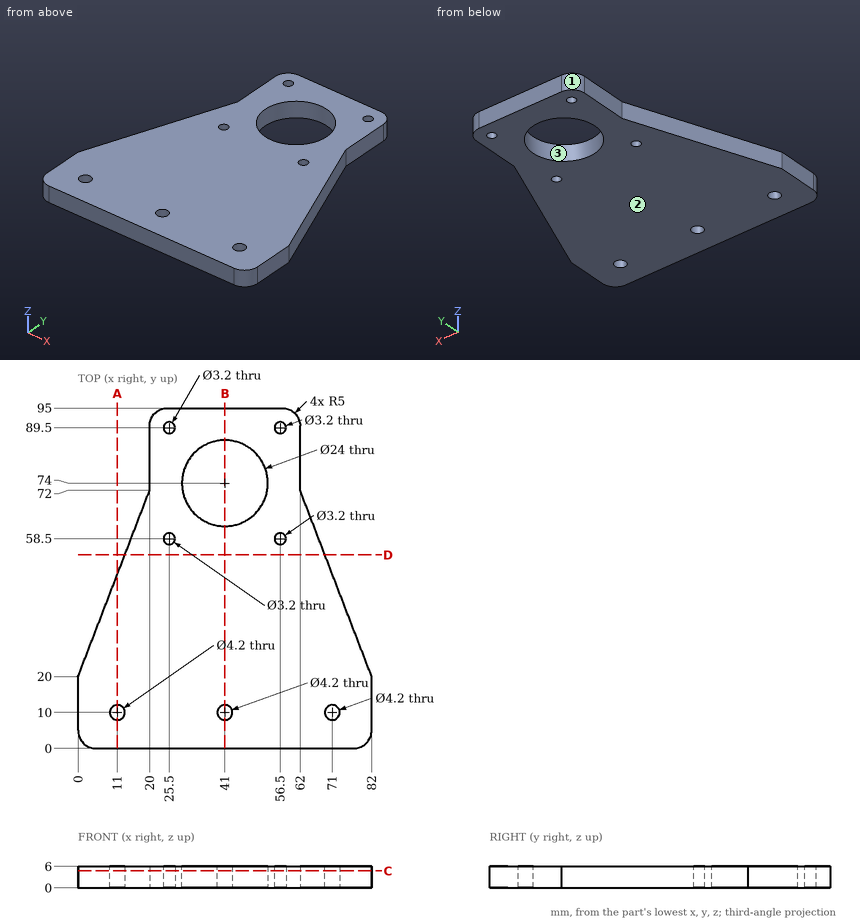
Here's the drawing with two shaded views (mm, measured from the low corner). I have some questions. Give positions to 0.01 mm unless a question says otherwise; leave off trailing zeros. Write each loop counter-clockwise with the first axis right and the second up, starting at its lowest first coordinate (ties: lowest second). Pieces come first, ordered by that corner, then holes. Notation, with made-up numbers: (55, -11) -> (82, -11) arc R21 cw to (82, 3) -> close; hole circle Ø7 at (4.25, 15.25). An arc over 180 degrees is marked (long way). Answer as a JSON object with one key per item and string values. Group by question number.
Item 1: Please list where these lines run through material, in increasing order: line 1 (Y direction, x = 25.5, z = 1.65); line 2 (X direction, y = 8.5, z = 5.25); line 3 (X direction, y = 65, z = 1.5) (1 decimal). Write a range as [from, to].
Item 2: Suppose I cut it at C-C (z = 4.75). State how many separate pieces and enclosed holes the cut face has, plus the area to 3 significant figures.
Item 3: We'd pull the mould along X, two halves only. Please class the marked faces 1, 2 and 3: +X half, -X half, draft (parallel to the pull), parting line (faces both ways), or undercut.
Item 4: Suppose I cut it at D-D (y = 54). Please give me the cut outline in (x, z), plus the area to 3 significant figures.
Item 5: Suppose I cut it at A-A (x = 11). Please give me the cut outline in (y, z).
Item 6: Suppose I cut it at B-B (x = 41). Please give me the cut outline in (y, z), plus the area to 3 significant figures.
Item 7: I'm going to push flat-ended pins straight in: P1, Ø1, axis at y = 31, z = 1, coming from the +X side; P2, Ø1.5, axis at y = 79.5, z = 4.5, coming from the -X side; P3, Ø1.8, axis at y = 77, z = 1.5, coming from the +X side. Where does each tip first touch, or does it pass through?
Findings:
{
 "1": {"line 1": "y = [0, 56.9], [60.1, 87.9], [91.1, 95]", "line 2": "x = [0, 9.53], [12.47, 39.53], [42.47, 69.53], [72.47, 82]", "line 3": "x = [17.3, 33.1], [48.9, 64.7]"},
 "2": {"separate pieces": "1", "enclosed holes": "8", "area": "5,280 mm²"},
 "3": {"face 1": "-X half", "face 2": "draft", "face 3": "undercut"},
 "4": {"outline": "(13.08, 0) -> (68.92, 0) -> (68.92, 6) -> (13.08, 6) -> close", "area": "335 mm²"},
 "5": {"outline": "(0, 0) -> (7.9, 0) -> (7.9, 6) -> (0, 6) -> close; (12.1, 0) -> (48.6, 0) -> (48.6, 6) -> (12.1, 6) -> close"},
 "6": {"outline": "(0, 0) -> (7.9, 0) -> (7.9, 6) -> (0, 6) -> close; (12.1, 0) -> (62, 0) -> (62, 6) -> (12.1, 6) -> close; (86, 0) -> (95, 0) -> (95, 6) -> (86, 6) -> close", "area": "401 mm²"},
 "7": {"P1": "stops at x = 77.96", "P2": "stops at x = 20", "P3": "stops at x = 62"}
}
